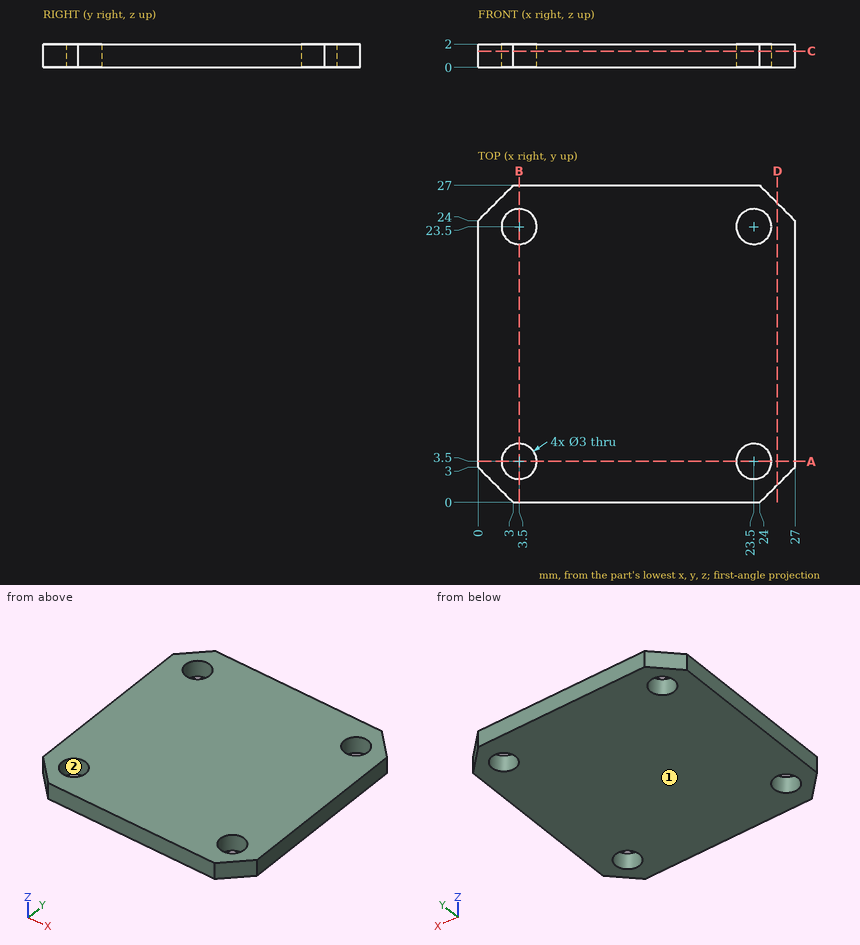
Design review of the part shown in the three views and the two pictorial views. Dimensions are in mm from the part's minimum x, y and z. Round coordinates to 2 decimals unless told otherwise and drop trailing zeros. Loops run counter-clockwise (first coordinate to the right, second up) from the corner with the lowest first, then second, coordinate; pieces in that order, holes last. Notation, with made-up numbers: M 68,2 L 117,2 A31 ccw 117,37 Z; hole C 66,10 d2. An arc over 180 degrees is marked long. Put each result on its own line as item: value.
Q1. Mouldability with a two-part tool opening along Y and no side actions: class the marked faces 1 and 2 as released by +Y, released by -Y, zero draft, split by the parting line, or undercut.
Result set:
face 1: zero draft
face 2: undercut
Q2. Consider section A-A, the plane y = 3.5. Give the boundary of the cut face in (x, z).
Result set:
outline: M 0,0 L 2,0 L 2,2 L 0,2 Z; M 5,0 L 22,0 L 22,2 L 5,2 Z; M 25,0 L 27,0 L 27,2 L 25,2 Z
Q3. To check wall thickness, follow L1, parallel to Y at x = 3.5, z = 1.05; L2, parallel to X at y = 4.5, z = 1.1; L3, parallel to Y at x = 2.75, z = 0.85. State the ranges of each line that lie inside material, in increasing order.
Result set:
L1: y = 0 to 2, 5 to 22, 25 to 27
L2: x = 0 to 2.38, 4.62 to 22.38, 24.62 to 27
L3: y = 0.25 to 2.2, 4.8 to 22.2, 24.8 to 26.75
Q4. Consider section C-C, the plane z = 1.4. Give the boundary of the cut face in (x, y).
Result set:
outline: M 0,3 L 3,0 L 24,0 L 27,3 L 27,24 L 24,27 L 3,27 L 0,24 Z; hole C 3.5,3.5 d3; hole C 3.5,23.5 d3; hole C 23.5,3.5 d3; hole C 23.5,23.5 d3
Q5. Consider section D-D, the plane x = 25.5. Give the boundary of the cut face in (y, z), then the cut area to 3 significant figures.
Result set:
outline: M 1.5,0 L 25.5,0 L 25.5,2 L 1.5,2 Z
area: 48.0 mm²
Q6. For pin 1 (1.8 mm diameter, centred on x = 3.5, y = 3.5, fed in from -Z), flat-tipped, find the tip position at first contact; note if it passes through.
Result set:
pin 1: passes through
